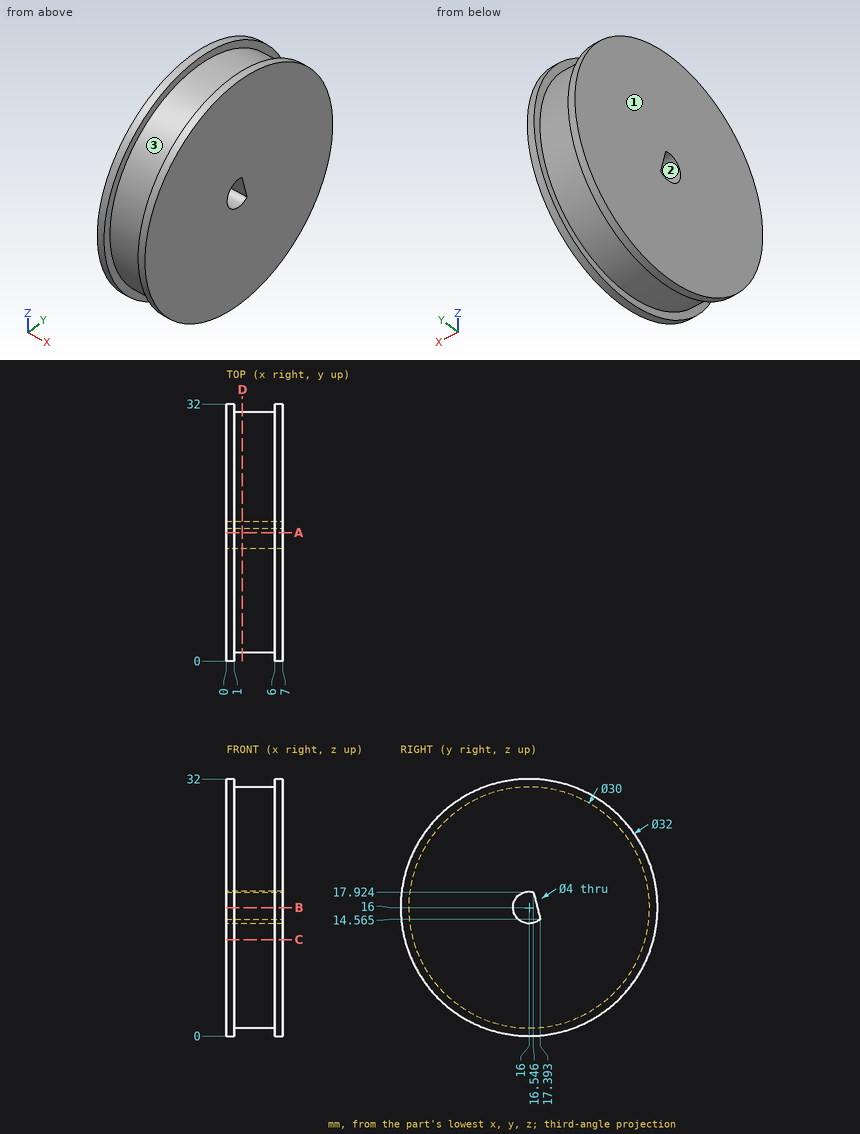
Could you check a few things on this drawing? It's one solid part, dimensions in mm from its lowest x, y, z. Give positions to 0.01 mm unless a question says otherwise; leave off trailing zeros. Write each loop counter-clockwise with the first axis right and the second up, starting at its lowest first coordinate (ties: lowest second). Pieces come first, ordered by that corner, then holes. Notation, with made-up numbers: M 37,57 L 56,57 A11 ccw 56,68 Z; hole C 0,39 d1. An arc over 180 degrees is marked long. Put each result on its own line as item: value. Start each with the question number.
Item 1: If we section it at A-A, the plane y = 16: Write out the boundary of the cut face in (x, z).
Item 2: If we section it at C-C, the plane z = 12: Write out the boundary of the cut face in (x, y).
Item 3: Will these pins go through, and if not, where does the flat tip stop? pin 1 (4 mm diameter, centred on x = 2, z = 13, fed in from +Y); pin 2 (1 mm diameter, centred on x = 4, z = 15.5, fed in from +Y); pin 3 (4 mm diameter, centred on x = 1, z = 18.5, fed in from -Y).
Item 4: If we section it at D-D, the plane x = 2: Write out the boundary of the cut face in (y, z) (1 decimal), then the cut area to 3 significant figures.
Item 5: If we section it at B-B, the plane z = 16: Write out the boundary of the cut face in (x, y).
Item 6: Thinking about a two-plate mould opening in Z: for the marked faces 1, 2 and 3, which applies, +Z half, -Z half, draft (parallel to the pull), parting line (faces both ways), or undercut?
Item 7: I need wall thicknesses on L1, parallel to X at y = 7, z = 3.5; L2, parallel to Y at x = 3, z = 16; L3, parallel to Z at x = 4.75, y = 18. Which ranges of each line are inside material? Lowest first, please. Write a range as from..to.
Values:
1. outline: M 0,0 L 1,0 L 1,1 L 6,1 L 6,0 L 7,0 L 7,14 L 0,14 Z; M 0,18 L 7,18 L 7,32 L 6,32 L 6,31 L 1,31 L 1,32 L 0,32 Z
2. outline: M 0,0.51 L 1,0.51 L 1,1.54 L 6,1.54 L 6,0.51 L 7,0.51 L 7,31.49 L 6,31.49 L 6,30.46 L 1,30.46 L 1,31.49 L 0,31.49 Z
3. pin 1: y = 31.95
3. pin 2: y = 31
3. pin 3: y = 0.01
4. outline: C 16,16 d30; hole M 16.5,17.9 A2 ccw long 17.4,14.6 Z
4. area: 697 mm²
5. outline: M 0,0 L 1,0 L 1,1 L 6,1 L 6,0 L 7,0 L 7,14 L 0,14 Z; M 0,17.03 L 7,17.03 L 7,32 L 6,32 L 6,31 L 1,31 L 1,32 L 0,32 Z
6. face 1: draft
6. face 2: undercut
6. face 3: parting line
7. L1: 0..1, 6..7
7. L2: 1..14, 17.03..31
7. L3: 1.13..30.87
